Design review of the part built by this model. Coordinates are the model's own, in mm. A direction names the side the tool comes from. Coordinates: 2 decimals unless noted, no trailing zeros. Write each loop counter-clockwise with the first axis right and the second up, starting at its lowest first coordinate (ties: lowest second). Pieces come first, ordered by that corner, then holes.
Q1. Add section A-A, the plane y = 0. Give the boundary of the cut face in (x, z).
Q2. Machinability: for faces 4 (the face through (104, 4.5, 4)), 5 (the face through (52.554, -3.905, 5.367)), which of the approach directions +Z, -Z, +X, -X, +Y, -Y give a long, thin tool a straight path to every point of the face, cutting with its end or side? Answer none if there is none.
Q3. The part is to be moulded in two halves that separate along Y. For faces 1 (the face through (105, -4.5, 4)), 2 (the face through (107.669, 0.526, 4.437)), 3 (the face through (0, -2, 0)), say which applies: +Y half, -Y half, draft (parallel to the pull), parting line (faces both ways), or undercut.
Q4. Add section C-C, the plane x = 13. Give the boundary of the cut face in (y, z), plus the area to 3 significant figures.
Q5. Clearance check with flat-ended pins moving along their axes: pin 1 Ø1.5 at (y, z) = (-1, 2) entering from -X; pin 2 Ø1.5 at (y, z) = (-2.5, 6.5) entering from -X; pin 3 Ø1 at (y, z) = (-0.5, 1.5) entering from +X. State where each tip first meets the part, or that it passes through.
Q6. To check wall thickness, follow probe 1 along X at (y, z) = (-0.25, 7); probe 2 along X at (y, z) = (1, 5.25); probe 3 along X at (y, z) = (4, 5.5). State the ranges of each line that lie inside material, in increasing order.
Q7. Add section B-B, the plane z = 4.5. Give the boundary of the cut face in (x, y).
from build123d import *

# Parameters (mm, degrees)
SKETCH5_R           = 1.75
BOSS_EXTRUDE3_DEPTH = 9
CUT_EXTRUDE2_START  = 3.5
SKETCH7_R           = 7.5
SKETCH7_R_2         = 4
CUT_EXTRUDE2_DEPTH  = 99.5


with BuildPart() as part:
    # Sketch5 → Boss-Extrude3 (new body)
    with BuildSketch(Plane.XY):
        with BuildLine():
            Line((0, 4.5), (106, 4.5))
            ThreePointArc((106, 4.5), (110.5, 0), (106, -4.5))
            Line((106, -4.5), (0, -4.5))
            ThreePointArc((0, -4.5), (-4.5, 0), (0, 4.5))
        make_face()
        Circle(SKETCH5_R, mode=Mode.SUBTRACT)
        with Locations((106, 0)):
            Circle(SKETCH5_R, mode=Mode.SUBTRACT)
    extrude(amount=BOSS_EXTRUDE3_DEPTH)

    # Sketch7 → Cut-Extrude2 (cut)
    with BuildSketch(Plane(origin=(0, 0, 0), x_dir=(0, 0, -1), z_dir=(1, 0, 0)).offset(CUT_EXTRUDE2_START)):
        with Locations((-4.5, 0)):
            Circle(SKETCH7_R)
        with Locations((-4.5, 0)):
            Circle(SKETCH7_R_2, mode=Mode.SUBTRACT)
    extrude(amount=CUT_EXTRUDE2_DEPTH, mode=Mode.SUBTRACT)


solid = part.part
Here are the results:
1. outline: (-4.5, 0) - (-1.75, 0) - (-1.75, 9) - (-4.5, 9) - close; (1.75, 0) - (3.5, 0) - (3.5, 0.5) - (103, 0.5) - (103, 0) - (104.25, 0) - (104.25, 9) - (103, 9) - (103, 8.5) - (3.5, 8.5) - (3.5, 9) - (1.75, 9) - close; (107.75, 0) - (110.5, 0) - (110.5, 9) - (107.75, 9) - close
2. face 4: +Z, -Z, +X, -X, +Y
2. face 5: none
3. face 1: -Y half
3. face 2: undercut
3. face 3: draft
4. outline: circle Ø8 at (0, 4.5)
4. area: 50.3 mm2
5. pin 1: stops at x = -4.49
5. pin 2: stops at x = -4.15
5. pin 3: stops at x = 110.5
6. probe 1: x = -4.49 to -1.73, 1.73 to 104.27, 107.73 to 110.49
6. probe 2: x = -4.39 to -1.44, 1.44 to 104.56, 107.44 to 110.39
6. probe 3: x = -2.06 to 3.5, 103 to 108.06
7. outline: (0, -4.5) - (3.5, -4.5) - (3.5, -4) - (103, -4) - (103, -4.5) - (106, -4.5) arc R4.5 ccw to (106, 4.5) - (103, 4.5) - (103, 4) - (3.5, 4) - (3.5, 4.5) - (0, 4.5) arc R4.5 ccw to start; hole circle Ø3.5 at (0, 0); hole circle Ø3.5 at (106, 0)
